Geometry: final body of the model. Coordinates: model frame, mm. Face numbers are marked on the shaded views. A direction names the side the tool comes from. Coordinates: 2 decimals unless noted, no trailing zeros. Write each loop counter-clockwise with the first axis right and the second up, starting at its lowest first coordinate (ties: lowest second). Pieces come first, ordered by that corner, then holes. Notation, with made-up numbers: M 37,18 L 93,18 A5 cw 93,24 Z; hole C -3,50.5 d2. An arc over 180 degrees is marked long. Write item = value, one per line. Start each with the question number.
Item 1: Reachability of the marked faces 1, 2, 3 and 4 from +Z, -Z, +X, -X, +Y, -Y: full face, straight path, thin tool, end or side. Return the list, or none.
Item 2: First-contact query: pin 1 Ø5 at (y, z) = (10, -57) entering from +X; pin 2 Ø8 at (y, z) = (13, -21) entering from +X; pin 3 Ø8 at (y, z) = (10.5, -50.5) entering from +X. Flat tips, straight axial feed; report the tip coordinate or a pass-through.
Item 3: Section A-A on y = 11.43. Output: boundary loops of the cut face in (x, z), plus the area to 3 significant figures.
Item 4: Section B-B on y = 1.25. Output: boundary loops of the cut face in (x, z).
Item 5: Section C-C on x = 50.5. Output: boundary loops of the cut face in (y, z).
Item 6: Ray query, L1, parallel to Z at x = 27.7, y = 11.43; L2, parallel to Z at x = 28.7, y = 11.43; L3, parallel to X at y = 16, z = -5. Return the intervals inside material, ascending. Write a range as [from, to].
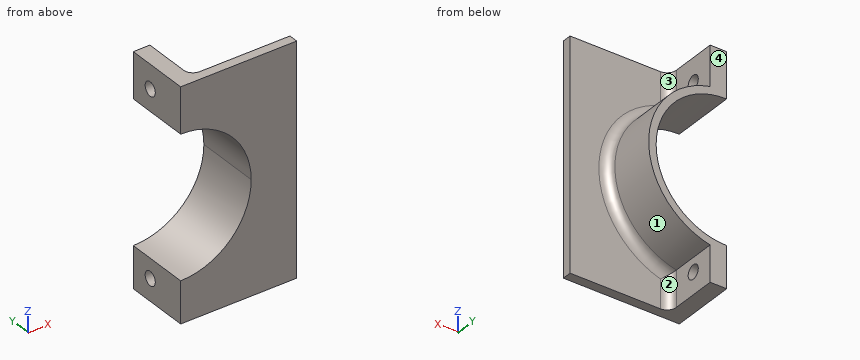
from build123d import *

# Parameters (mm, degrees)
BOSS_EXTRUDE12_DEPTH    = 17.78
BOSS_EXTRUDE13_DEPTH    = 2.54
FILLET2_R               = 2.54
SKETCH5_R               = 1.905
CUT_EXTRUDE1_DEPTH      = 58.15
CUT_EXTRUDE1_DEPTH_BACK = 1


with BuildPart() as part:
    # Sketch3 → Boss-Extrude12 (new body)
    with BuildSketch(Plane(origin=(0, 0, 0), x_dir=(1, 0, 0), z_dir=(0, 1, 0))):
        with BuildLine():
            Line((25.4, 12.446), (25.4, 0))
            Line((25.4, 0), (29.929832056, 0))
            Line((29.929832056, 0), (29.929832056, 10.900407257))
            ThreePointArc((29.929832056, 10.900407257), (46.736, 31.75), (29.929832056, 52.599592743))
            Line((29.929832056, 52.599592743), (29.929832056, 62.41624918))
            Line((29.929832056, 62.41624918), (25.4, 62.41624918))
            Line((25.4, 62.41624918), (25.4, 51.054))
            ThreePointArc((25.4, 51.054), (39.049989304, 45.399989304), (44.704, 31.75))
            ThreePointArc((44.704, 31.75), (39.049989304, 18.100010696), (25.4, 12.446))
        make_face()
    extrude(amount=BOSS_EXTRUDE12_DEPTH)

    # Sketch3<16> → Boss-Extrude13 (add)
    with BuildSketch(Plane(origin=(0, 0, 0), x_dir=(1, 0, 0), z_dir=(0, 1, 0))):
        with BuildLine():
            Line((29.929832056, 10.900407257), (29.929832056, 0))
            Line((29.929832056, 0), (57.15, 0))
            Line((57.15, 0), (57.15, 62.41624918))
            Line((57.15, 62.41624918), (29.929832056, 62.41624918))
            Line((29.929832056, 62.41624918), (29.929832056, 52.599592743))
            ThreePointArc((29.929832056, 52.599592743), (46.736, 31.75), (29.929832056, 10.900407257))
        make_face()
    extrude(amount=BOSS_EXTRUDE13_DEPTH)

    # Fillet2
    fillet2_edges = [part.edges().sort_by_distance(p)[0] for p in [
        (46.736, 2.54, -31.75),
        (29.929832056, 2.54, -5.450203629),
        (29.929832056, 2.54, -57.507920962),
    ]]
    fillet(fillet2_edges, radius=FILLET2_R)

    # Sketch5 → Cut-Extrude1 (cut, two sides)
    with BuildSketch(Plane(origin=(0, 0, 0), x_dir=(0, 0, -1), z_dir=(1, 0, 0))) as cut_extrude1_sk:
        with Locations((6.5405, 11.43)):
            Circle(SKETCH5_R)
        with Locations((56.41762459, 11.43)):
            Circle(SKETCH5_R)
    extrude(amount=CUT_EXTRUDE1_DEPTH, mode=Mode.SUBTRACT)
    extrude(cut_extrude1_sk.sketch, amount=-CUT_EXTRUDE1_DEPTH_BACK, mode=Mode.SUBTRACT)


solid = part.part
Responses:
q1.face_1 = +X, +Y
q1.face_2 = -Z, +X, +Y
q1.face_3 = +Z, +X, +Y
q1.face_4 = +Z, -Z, +X, -X, +Y
q2.pin_1 = 29.93
q2.pin_2 = 45.64
q2.pin_3 = 40.82
q3.outline = M 25.4,-62.42 L 29.93,-62.42 L 29.93,-58.32 L 25.4,-58.32 Z; M 25.4,-54.51 L 29.93,-54.51 L 29.93,-52.6 A21.34 ccw 29.93,-10.9 L 29.93,-8.45 L 25.4,-8.45 L 25.4,-12.45 A19.3 cw 25.4,-51.05 Z; M 25.4,-4.64 L 29.93,-4.64 L 29.93,0 L 25.4,0 Z
q3.area = 186 mm²
q4.outline = M 25.4,-62.42 L 57.15,-62.42 L 57.15,0 L 25.4,0 L 25.4,-12.45 A19.3 cw 25.4,-51.05 Z
q5.outline = M 0,-62.42 L 2.54,-62.42 L 2.54,0 L 0,0 Z
q6.L1 = [-62.42, -58.32], [-54.51, -50.92], [-12.58, -8.45], [-4.64, 0]
q6.L2 = [-62.42, -58.32], [-54.51, -50.77], [-12.73, -8.45], [-4.64, 0]
q6.L3 = [25.4, 29.93]
